Can you work these out from the drawing? Everything is in mm from the part's minimum corner. Give positions to 0.01 mm unless a question says otherwise; leave off trailing zeros. Loops run counter-clockwise (first coordinate to the right, second up) from the corner with the lowest first, then second, coordinate; pieces in that order, holes last. Notation, with made-up numbers: M -7.75,37.25 L 29.25,37.25 A27 cw 29.25,63.25 Z; hole C 77.5,-11.75 d3. An arc over 180 degrees is marked long. Use CSV: the item, a comma, the result in double quotes.
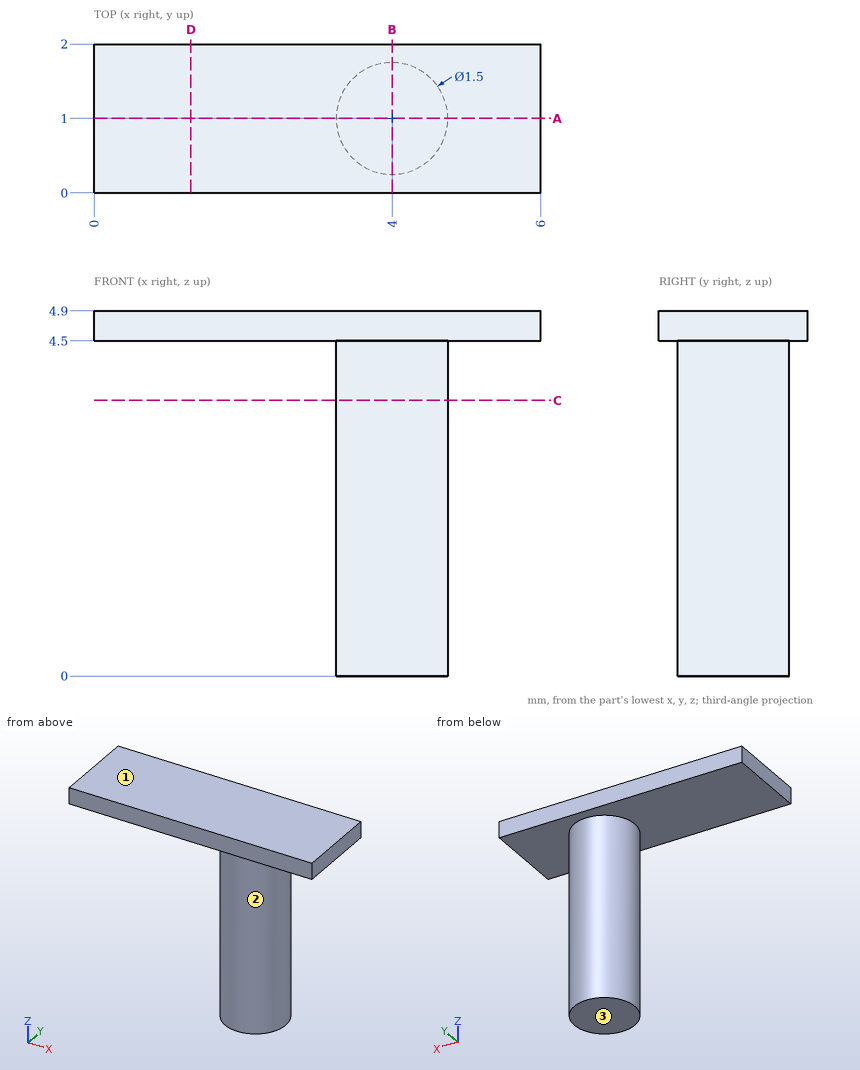
Q1. I want a section at C-C, the plane z = 3.7. Please give me the cut outline in (x, y), then the cut area to 3 significant figures.
Model answer:
outline,"C 4,1 d1.5"
area,"1.77 mm2"
Q2. I want a section at B-B, the plane x = 4. Please give me the cut outline in (y, z), then the cut area to 3 significant figures.
Model answer:
outline,"M 0,4.5 L 0.25,4.5 L 0.25,0 L 1.75,0 L 1.75,4.5 L 2,4.5 L 2,4.9 L 0,4.9 Z"
area,"7.55 mm2"
Q3. If we mould it in two halves opening along Z, with no side actions, what happens to the marked faces 1, 2 and 3? For each: released by +Z, released by -Z, zero draft, split by the parting line, or undercut.
Model answer:
face 1,"released by +Z"
face 2,"zero draft"
face 3,"released by -Z"
Q4. Please list where these lines run through material, in increasing order: L1, parallel to Z at x = 1.55, y = 1.5; L2, parallel to X at y = 1.4, z = 1.7; L3, parallel to X at y = 0.4, z = 3.55. Write a range as from..to.
Model answer:
L1,"4.5..4.9"
L2,"3.37..4.63"
L3,"3.55..4.45"
Q5. I want a section at A-A, the plane y = 1. Please give me the cut outline in (x, z).
Model answer:
outline,"M 0,4.5 L 3.25,4.5 L 3.25,0 L 4.75,0 L 4.75,4.5 L 6,4.5 L 6,4.9 L 0,4.9 Z"
Q6. I want a section at D-D, the plane x = 1.3. Please give me the cut outline in (y, z).
Model answer:
outline,"M 0,4.5 L 2,4.5 L 2,4.9 L 0,4.9 Z"
